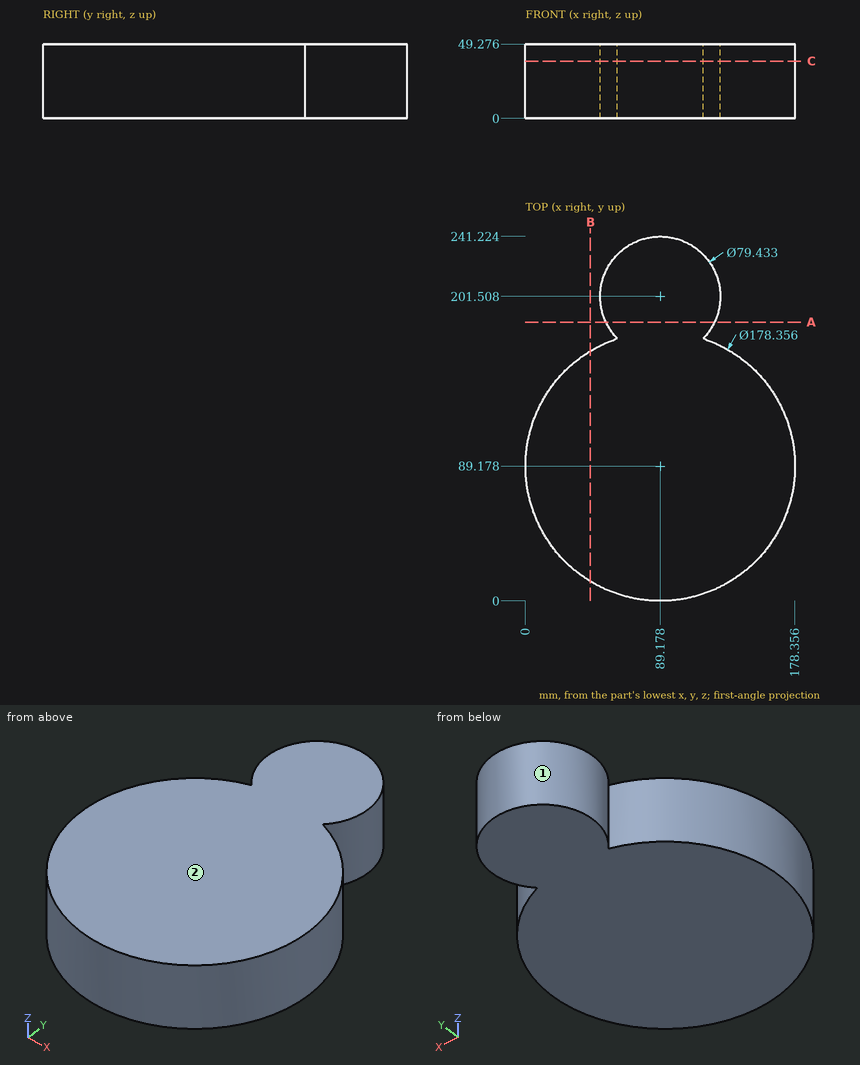
Design review of the part shown in the three views and the two pictorial views. Dimensions are in mm from the part's minimum x, y and z. Round coordinates to 2 decimals unless told otherwise and drop trailing zeros. Write each loop counter-clockwise with the first axis right and the second up, starting at its lowest first coordinate (ties: lowest second). Pieces come first, ordered by that corner, then holes. Notation, with made-up numbers: (-32.5, 42) -> (-4.5, 42) arc R21 ccw to (-4.5, 68) -> close; hole circle Ø10 at (57, 20.25). An arc over 180 degrees is marked (long way). Write item = value, one per line. Start each with the question number.
1) Wall thickness on probe 1 along Y at (x, z) = (44, 6.5) (1 decimal); probe 2 along Y at (x, z) = (106.5, 13.5); probe 3 along X at (y, z) = (107, 37): over which ranges is each line inside the solid? List them lowest first. Write a range as from..to.
2) Take a section at C-C, the plane z = 38. State the section outline as (x, y) points.
3) Mouldability with a two-part tool opening along Y and no side actions: class the marked faces 1 and 2 as +Y half, -Y half, draft (parallel to the pull), parting line (faces both ways), or undercut.
4) Take a section at A-A, the plane y = 184.5. State the section outline as (x, z) points, plus the area to 3 significant figures.
5) Clearance check with flat-ended pins moving along their axes: pin 1 (1 mm diameter, centred on y = 208, z = 22.5, fed in from +X); pin 2 (1.5 mm diameter, centred on x = 150, z = 7, fed in from -Y); pin 3 (12 mm diameter, centred on y = 25.5, z = 28.5, fed in from -X) (1 decimal). State where each tip first meets the part, or that it passes through.
6) Take a section at B-B, the plane x = 43. State the section outline as (y, z) points.
Results list:
q1.probe_1 = 12.3..166.1
q1.probe_2 = 1.7..237.25
q1.probe_3 = 1.8..176.56
q2.outline = (60.8, 173.72) arc R89.18 ccw (long way) to (117.56, 173.72) arc R39.72 ccw (long way) to start
q3.face_1 = undercut
q3.face_2 = draft
q4.outline = (53.29, 0) -> (125.07, 0) -> (125.07, 49.28) -> (53.29, 49.28) -> close
q4.area = 3,540 mm²
q5.pin_1 = 128.44
q5.pin_2 = 23.27
q5.pin_3 = 21.2
q6.outline = (12.89, 0) -> (165.47, 0) -> (165.47, 49.28) -> (12.89, 49.28) -> close
